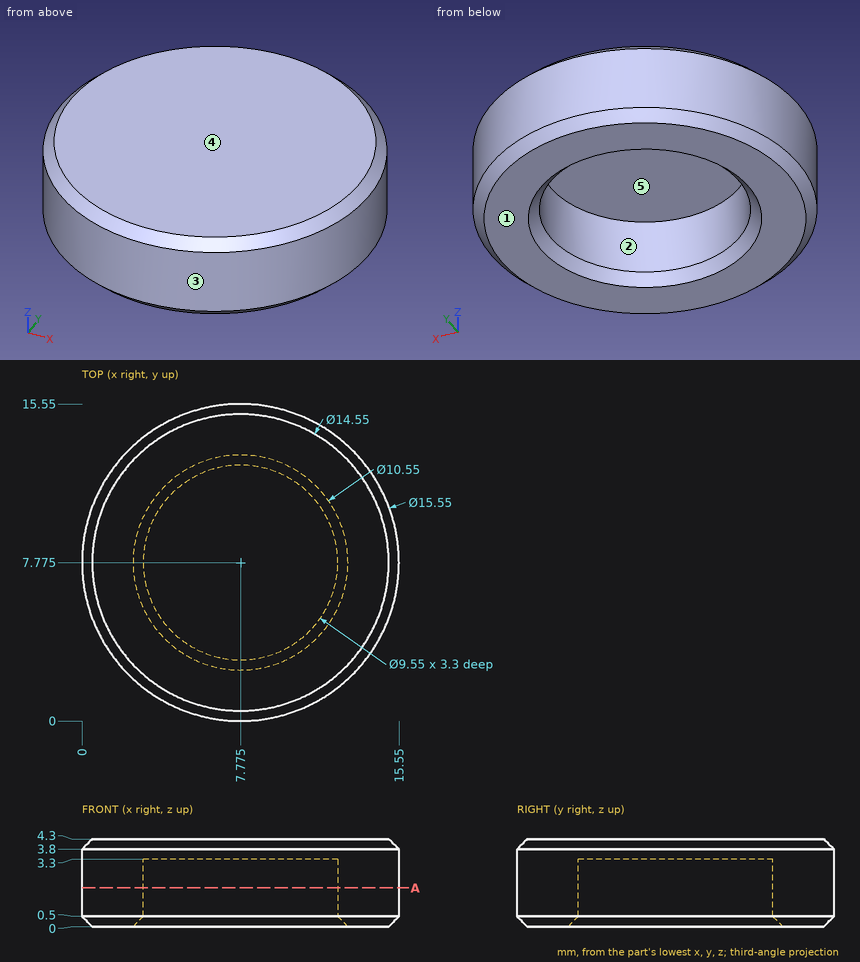
Geometry check sheet. Reference: drawing and pictorial views, mm from the part's lowest x, y, z. A direction names the side the tool comes from. Round coordinates to 2 decimals unless told otherwise and drop trailing zeros. Order: outer loops, then holes, each group sorted by start corner. A loop starts at its lowest first (then second) coordinate and runs counter-clockwise, first axis right, second up. Notation, with made-up numbers: (87.5, 6.25) - (124.5, 6.25) arc R24 cw to (124.5, 16.25) - close; hole circle Ø1 at (10, 86.5). An arc over 180 degrees is marked (long way). One line per question, with ' | ' between items. Start each with the question number.
(1) Release check for a two-part mould opening along X. For the marked faces 3, 4 and 5 record: released by +X, released by -X, zero draft, split by the parting line, or undercut.
(2) Depth check by flat-ended pin: pin 1 Ø1 at (x, z) = (8.5, 2.5) entering from -Y; pin 2 Ø1 at (y, z) = (9, 1) entering from -X; pin 3 Ø1 at (x, z) = (13, 1) entering from -Y. Enter the tip coordinate at first touch or a pass-through.
(3) Thickness scan on L1, parallel to X at y = 9.5, z = 3; L2, parallel to X at y = 7, z = 2.2; L3, parallel to Z at x = 7, y = 8.5. Record the ranges inside material, lowest first. Write a range as [from, to].
(4) Sectioned sample at A-A on z = 1.9. Record the cut outline in (x, y) (3 decimals).
(5) Access from +Z, -Z, +X, -X, +Y, -Y to the whole of each face (thin tool, end or side, straight path). Record for the marked faces 1 and 2.
Conclusion:
1) face 3: split by the parting line | face 4: zero draft | face 5: undercut
2) pin 1: stops at y = 0 | pin 2: stops at x = 0.03 | pin 3: stops at y = 1.6
3) L1: x = [0.19, 3.32], [12.23, 15.36] | L2: x = [0.04, 3.06], [12.49, 15.51] | L3: z = [3.3, 4.3]
4) outline: circle Ø15.55 at (7.775, 7.775); hole circle Ø9.55 at (7.775, 7.775)
5) face 1: -Z, +X, -X, +Y, -Y | face 2: -Z
